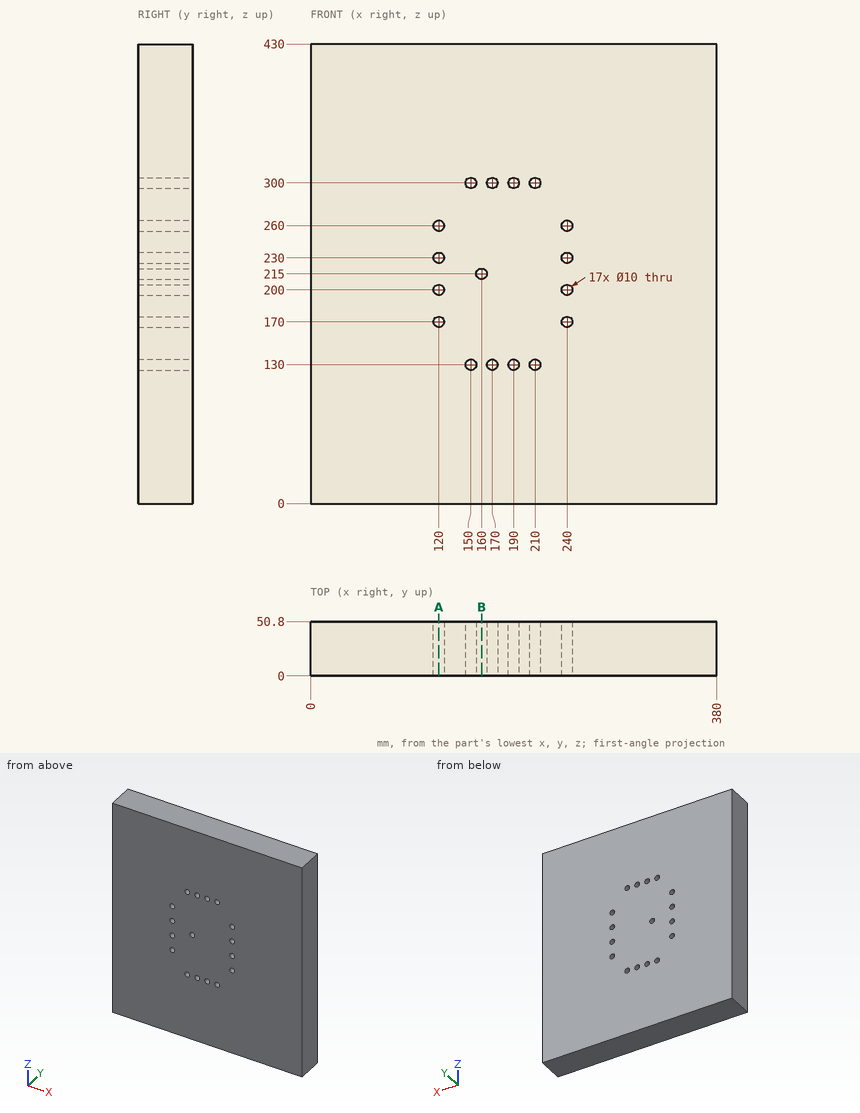
Job drawing, mm, ordinate dimensions from the low corner. One solid piece. Give positions to 0.01 mm unless a question says otherwise; leave off trailing zeros. Write each loop counter-clockwise with the first axis right and the second up, starting at its lowest first coordinate (ties: lowest second). Pieces come first, ordered by that corner, then holes. Notation, with made-up numbers: M 5,82.25 L 17,82.25 A21 cw 17,113.25 Z; hole C 23.25,73 d6. An arc over 180 degrees is marked long. One line per item, written item: value. Start each with the question number.
Q1. Probe probe 1 along X at (y, z) = (37, 300); probe 2 along X at (y, z) = (32.5, 170); probe 3 along Z at (x, y) = (170, 12.5). List the from-to ranges inside material, lowest first. Write a range as [from, to].
Q2. Saw through at B-B, the plane x = 160. Write the cut outline in (y, z).
Q3. Saw through at A-A, the plane x = 120. Write the cut outline in (y, z).
Output values:
1. probe 1: x = [0, 145], [155, 165], [175, 185], [195, 205], [215, 380]
1. probe 2: x = [0, 115], [125, 235], [245, 380]
1. probe 3: z = [0, 125], [135, 295], [305, 430]
2. outline: M 0,0 L 50.8,0 L 50.8,210 L 0,210 Z; M 0,220 L 50.8,220 L 50.8,430 L 0,430 Z
3. outline: M 0,0 L 50.8,0 L 50.8,165 L 0,165 Z; M 0,175 L 50.8,175 L 50.8,195 L 0,195 Z; M 0,205 L 50.8,205 L 50.8,225 L 0,225 Z; M 0,235 L 50.8,235 L 50.8,255 L 0,255 Z; M 0,265 L 50.8,265 L 50.8,430 L 0,430 Z
